Verification items for the finished model (mm, model axes). Coordinates: 2 decimals unless noted, no trailing zeros. Order: outer loops, then holes, each group sorted by start corner. A loop starts at its lowest first (then second) coordinate and runs counter-clockwise, first axis right, second up. Notation, with made-up numbers: (13, 14.5) -> (41, 14.5) arc R19 cw to (41, 29.5) -> close; hole circle Ø7 at (-31, 38.25). An arc over 180 degrees is marked (long way). Write item = value, one per line. Start each with the question number.
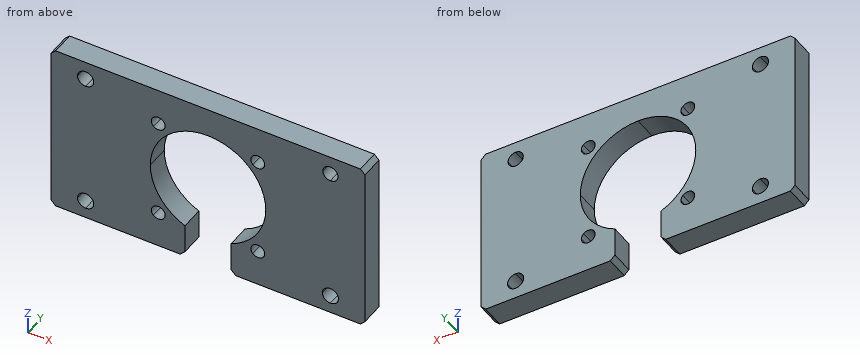
from build123d import *

# Parameters (mm, degrees)
F1_DEPTH = 10


# Not quite as in the source:
# - ends of sketch curves that miss each other by under 0.0002 mm in the source are joined


with BuildPart() as f1:
    # F0 (on Front) → F1 (new body)
    with BuildSketch(Plane.XZ):
        with BuildLine():
            Line((-28.537618, -30.289698), (25.462382, -30.289698))
            Line((25.462382, -30.289698), (27.462382, -28.289698))
            Line((27.462382, -28.289698), (27.462382, 42.710302))
            Line((27.462382, 42.710302), (25.462382, 44.710302))
            Line((25.462382, 44.710302), (-106.537618, 44.710302))
            Line((-106.537618, 44.710302), (-108.537618, 42.710302))
            Line((-108.537618, 42.710302), (-108.537618, -28.289698))
            Line((-108.537618, -28.289698), (-106.537618, -30.289698))
            Line((-106.537618, -30.289698), (-52.537618, -30.289698))
            Line((-52.537618, -30.289698), (-50.537618, -28.289698))
            Line((-50.537618, -28.289698), (-50.537618, -21.6037570684))
            ThreePointArc((-50.537618, -21.6037570684), (-55.4409257201, -19.4006246843), (-59.881294185, -16.3708809994))
            ThreePointArc((-59.881294185, -16.3708809994), (-62.0305817628, -17.3555463136), (-64.2256943436, -16.4777743436))
            ThreePointArc((-64.2256943436, -16.4777743436), (-65.1034663136, -14.2826617628), (-64.1188009994, -12.133374185))
            ThreePointArc((-64.1188009994, -12.133374185), (-69.2558707453, -3.0615994432), (-71.037618, 7.210302))
            ThreePointArc((-71.037618, 7.210302), (-69.2558706203, 17.4822037925), (-64.1188005289, 26.5539787586))
            ThreePointArc((-64.1188005289, 26.5539787586), (-65.1034663058, 28.7032664454), (-64.2256943436, 30.8983793436))
            ThreePointArc((-64.2256943436, 30.8983793436), (-62.0305813759, 31.7761513041), (-59.8812936652, 30.7914854258))
            ThreePointArc((-59.8812936652, 30.7914854258), (-50.8095191267, 35.9285548585), (-40.537618, 37.710302))
            ThreePointArc((-40.537618, 37.710302), (-30.265716524, 35.9285547335), (-21.1939417612, 30.7914849552))
            ThreePointArc((-21.1939417612, 30.7914849552), (-19.0446539415, 31.7761512963), (-16.8495406564, 30.8983793436))
            ThreePointArc((-16.8495406564, 30.8983793436), (-16.1992224025, 29.9251092971), (-15.970861, 28.777059))
            ThreePointArc((-15.970861, 28.777059), (-16.2283003475, 27.5611802778), (-16.9564350448, 26.5539782388))
            ThreePointArc((-16.9564350448, 26.5539782388), (-11.8193652665, 17.482203476), (-10.037618, 7.210302))
            ThreePointArc((-10.037618, 7.210302), (-11.8193651415, -3.0615991267), (-16.9564345742, -12.1333736652))
            ThreePointArc((-16.9564345742, -12.1333736652), (-16.2283002188, -13.140575568), (-15.970861, -14.356454))
            ThreePointArc((-15.970861, -14.356454), (-16.1992224025, -15.5045042971), (-16.8495406564, -16.4777743436))
            ThreePointArc((-16.8495406564, -16.4777743436), (-19.0446535546, -17.3555463058), (-21.1939412414, -16.3708805289))
            ThreePointArc((-21.1939412414, -16.3708805289), (-25.6343099562, -19.4006245031), (-30.537618, -21.6037570684))
            Line((-30.537618, -21.6037570684), (-30.537618, -28.289698))
            Line((-30.537618, -28.289698), (-28.537618, -30.289698))
        make_face()
        with BuildLine():
            ThreePointArc((-93.537618, -18.789698), (-91.0627442658, -19.8148242658), (-90.037618, -22.289698))
            ThreePointArc((-90.037618, -22.289698), (-91.0627442658, -24.7645717342), (-93.537618, -25.789698))
            ThreePointArc((-93.537618, -25.789698), (-96.0124917342, -24.7645717342), (-97.037618, -22.289698))
            ThreePointArc((-97.037618, -22.289698), (-96.0124917342, -19.8148242658), (-93.537618, -18.789698))
        make_face(mode=Mode.SUBTRACT)
        with BuildLine():
            ThreePointArc((12.462382, -18.789698), (14.9372557342, -19.8148242658), (15.962382, -22.289698))
            ThreePointArc((15.962382, -22.289698), (14.9372557342, -24.7645717342), (12.462382, -25.789698))
            ThreePointArc((12.462382, -25.789698), (9.9875082658, -24.7645717342), (8.962382, -22.289698))
            ThreePointArc((8.962382, -22.289698), (9.9875082658, -19.8148242658), (12.462382, -18.789698))
        make_face(mode=Mode.SUBTRACT)
        with BuildLine():
            ThreePointArc((-93.537618, 40.210302), (-91.0627442658, 39.1851757342), (-90.037618, 36.710302))
            ThreePointArc((-90.037618, 36.710302), (-91.0627442658, 34.2354282658), (-93.537618, 33.210302))
            ThreePointArc((-93.537618, 33.210302), (-96.0124917342, 34.2354282658), (-97.037618, 36.710302))
            ThreePointArc((-97.037618, 36.710302), (-96.0124917342, 39.1851757342), (-93.537618, 40.210302))
        make_face(mode=Mode.SUBTRACT)
        with BuildLine():
            ThreePointArc((12.462382, 33.410302), (10.1289296221, 34.3768496221), (9.162382, 36.710302))
            ThreePointArc((9.162382, 36.710302), (10.1289296221, 39.0437543779), (12.462382, 40.010302))
            ThreePointArc((12.462382, 40.010302), (14.7958343779, 39.0437543779), (15.762382, 36.710302))
            ThreePointArc((15.762382, 36.710302), (14.7958343779, 34.3768496221), (12.462382, 33.410302))
        make_face(mode=Mode.SUBTRACT)
        with BuildLine():
            ThreePointArc((-40.537618, 32.210302), (-22.8599484703, 24.8879715297), (-15.537618, 7.210302))
            Line((-15.537618, 7.210302), (-10.037618, 7.210302))
            ThreePointArc((-10.037618, 7.210302), (-11.8193652665, 17.482203476), (-16.9564350448, 26.5539782388))
            ThreePointArc((-16.9564350448, 26.5539782388), (-19.0446539415, 25.7779667037), (-21.0921813436, 26.6557386564))
            ThreePointArc((-21.0921813436, 26.6557386564), (-21.9699532963, 28.7032660585), (-21.1939417612, 30.7914849552))
            ThreePointArc((-21.1939417612, 30.7914849552), (-30.265716524, 35.9285547335), (-40.537618, 37.710302))
            Line((-40.537618, 37.710302), (-40.537618, 32.210302))
        make_face()
        with BuildLine():
            ThreePointArc((-65.537618, 7.210302), (-58.2152875297, 24.8879715297), (-40.537618, 32.210302))
            Line((-40.537618, 32.210302), (-40.537618, 37.710302))
            ThreePointArc((-40.537618, 37.710302), (-50.8095191267, 35.9285548585), (-59.8812936652, 30.7914854258))
            ThreePointArc((-59.8812936652, 30.7914854258), (-59.3053347894, 29.8565864419), (-59.104374, 28.777059))
            ThreePointArc((-59.104374, 28.777059), (-59.3327354025, 27.6290087029), (-59.9830536564, 26.6557386564))
            ThreePointArc((-59.9830536564, 26.6557386564), (-62.0305814454, 25.7779666942), (-64.1188005289, 26.5539787586))
            ThreePointArc((-64.1188005289, 26.5539787586), (-69.2558706203, 17.4822037925), (-71.037618, 7.210302))
            Line((-71.037618, 7.210302), (-65.537618, 7.210302))
        make_face()
        with BuildLine():
            ThreePointArc((-59.881294185, -16.3708809994), (-55.4409257201, -19.4006246843), (-50.537618, -21.6037570684))
            Line((-50.537618, -21.6037570684), (-50.537618, -15.702576))
            ThreePointArc((-50.537618, -15.702576), (-61.4541187154, -6.4827618582), (-65.537618, 7.210302))
            Line((-65.537618, 7.210302), (-71.037618, 7.210302))
            ThreePointArc((-71.037618, 7.210302), (-69.2558707453, -3.0615994432), (-64.1188009994, -12.133374185))
            ThreePointArc((-64.1188009994, -12.133374185), (-62.0305817628, -11.3573616864), (-59.9830536564, -12.2351336564))
            ThreePointArc((-59.9830536564, -12.2351336564), (-59.3327354025, -13.2084037029), (-59.104374, -14.356454))
            ThreePointArc((-59.104374, -14.356454), (-59.3053349287, -15.435981803), (-59.881294185, -16.3708809994))
        make_face()
        with BuildLine():
            Line((-30.537618, -15.702576), (-30.537618, -21.6037570684))
            ThreePointArc((-30.537618, -21.6037570684), (-25.6343099562, -19.4006245031), (-21.1939412414, -16.3708805289))
            ThreePointArc((-21.1939412414, -16.3708805289), (-21.9699533058, -14.2826614454), (-21.0921813436, -12.2351336564))
            ThreePointArc((-21.0921813436, -12.2351336564), (-19.0446536241, -11.3573616959), (-16.9564345742, -12.1333736652))
            ThreePointArc((-16.9564345742, -12.1333736652), (-11.8193651415, -3.0615991267), (-10.037618, 7.210302))
            Line((-10.037618, 7.210302), (-15.537618, 7.210302))
            ThreePointArc((-15.537618, 7.210302), (-19.6211172846, -6.4827618582), (-30.537618, -15.702576))
        make_face()
    extrude(amount=-F1_DEPTH)


solid = f1.part
Item 1: Section check A-A (z = 38.5). Record the boundary of the cut face in (x, y), then the cut area to 3 significant figures.
Item 2: Thickness scan on line 1 (X direction, y = 6, z = 36.5); line 2 (Z direction, x = 15.5, y = 6.25); line 3 (Z direction, x = -90.5, y = 7). Record the ranges inside material, lowest first.
Item 3: Section check C-C (y = 3.75). State how many separate pieces and enclosed holes the cut face has, then the cut area to 3 significant figures.
Item 4: Section check B-B (z = 10). Record the boundary of the cut face in (x, y).
Filled sheet:
q1.outline = (-108.54, 0) -> (-96.55, 0) -> (-96.55, 10) -> (-108.54, 10) -> close; (-90.53, 0) -> (9.69, 0) -> (9.69, 10) -> (-90.53, 10) -> close; (15.23, 0) -> (27.46, 0) -> (27.46, 10) -> (15.23, 10) -> close
q1.area = 1,240 mm^2
q2.line_1 = -108.54 to -97.03, -90.04 to 9.17, 15.76 to 27.46
q2.line_2 = -30.29 to -24.03, -20.55 to 35.42, 38 to 44.71
q2.line_3 = -30.29 to -24.03, -20.55 to 34.97, 38.45 to 44.71
q3.separate_pieces = 1
q3.enclosed_holes = 8
q3.area = 7,700 mm^2
q4.outline = (-108.54, 0) -> (-65.38, 0) -> (-65.38, 10) -> (-108.54, 10) -> close; (-15.69, 0) -> (27.46, 0) -> (27.46, 10) -> (-15.69, 10) -> close
